```python
from build123d import *

# Parameters (mm, degrees)
CYLINDER039_R     = 68.3
CYLINDER039_DEPTH = 5
CYLINDER036_R     = 40
CYLINDER036_DEPTH = 27.4
CYLINDER035_R     = 45
CYLINDER035_DEPTH = 23.4
CYLINDER033_R     = 45
CYLINDER033_DEPTH = 25
CYLINDER032_R     = 48
CYLINDER032_DEPTH = 3.2
CYLINDER029_R     = 46.6
CYLINDER029_DEPTH = 6
CYLINDER038_R     = 46.6
CYLINDER038_DEPTH = 4
CYLINDER030_R     = 48
CYLINDER030_DEPTH = 4
CYLINDER037_R     = 48
CYLINDER037_DEPTH = 1.2
CYLINDER031_R     = 45
CYLINDER031_DEPTH = 25
CYLINDER034_R     = 51.3
CYLINDER034_DEPTH = 5
CHAMFER003_SIZE   = 1.2
CHAMFER002_SIZE   = 1.2


with BuildPart() as obj1:
    # Cylinder039 → Cylinder039 (new body)
    with BuildSketch(Plane.XY.offset(-23.2)):
        Circle(CYLINDER039_R)
    extrude(amount=CYLINDER039_DEPTH)


with BuildPart() as cone002:
    # Cone002 → Cone002 (revolve)
    with BuildSketch(Plane(origin=(0, 0, -15.2), x_dir=(-1, 0, 0), z_dir=(0, -1, 0))):
        Polygon((0, 0), (40, 0), (45, 5), (0, 5), align=None)
    revolve(axis=Axis((0, 0, -15.2), (0, 0, -1)))


with BuildPart() as fusion010:
    # Cylinder036 → Cylinder036 (new body)
    with BuildSketch(Plane.XY.offset(-17)):
        Circle(CYLINDER036_R)
    extrude(amount=CYLINDER036_DEPTH)

    # Fusion010: union Cone002
    add(cone002.part)


with BuildPart() as cut015:
    # Cylinder035 → Cylinder035 (new body)
    with BuildSketch(Plane.XY.offset(-20.2)):
        Circle(CYLINDER035_R)
    extrude(amount=CYLINDER035_DEPTH)

    # Cut015: cut Fusion010
    add(fusion010.part, mode=Mode.SUBTRACT)


with BuildPart() as cylinder033:
    # Cylinder033 → Cylinder033 (new body)
    with BuildSketch(Plane.XY.offset(-18)):
        Circle(CYLINDER033_R)
    extrude(amount=CYLINDER033_DEPTH)


with BuildPart() as cylinder032:
    # Cylinder032 → Cylinder032 (new body)
    with BuildSketch(Plane.XY):
        Circle(CYLINDER032_R)
    extrude(amount=CYLINDER032_DEPTH)


with BuildPart() as cylinder029:
    # Cylinder029 → Cylinder029 (new body)
    with BuildSketch(Plane.XY.offset(-14)):
        Circle(CYLINDER029_R)
    extrude(amount=CYLINDER029_DEPTH)


with BuildPart() as cylinder038:
    # Cylinder038 → Cylinder038 (new body)
    with BuildSketch(Plane.XY.offset(-4)):
        Circle(CYLINDER038_R)
    extrude(amount=CYLINDER038_DEPTH)


with BuildPart() as cylinder030:
    # Cylinder030 → Cylinder030 (new body)
    with BuildSketch(Plane.XY.offset(-8)):
        Circle(CYLINDER030_R)
    extrude(amount=CYLINDER030_DEPTH)


with BuildPart() as cut016:
    # Cylinder037 → Cylinder037 (new body)
    with BuildSketch(Plane.XY.offset(-15.2)):
        Circle(CYLINDER037_R)
    extrude(amount=CYLINDER037_DEPTH)

    # Fusion012: union Cylinder032, Cylinder029, Cylinder038, Cylinder030
    add(cylinder032.part)
    add(cylinder029.part)
    add(cylinder038.part)
    add(cylinder030.part)

    # Cut016: cut Cylinder033
    add(cylinder033.part, mode=Mode.SUBTRACT)


with BuildPart() as cylinder031:
    # Cylinder031 → Cylinder031 (new body)
    with BuildSketch(Plane.XY.offset(-23)):
        Circle(CYLINDER031_R)
    extrude(amount=CYLINDER031_DEPTH)


with BuildPart() as cut014:
    # Cylinder034 → Cylinder034 (new body)
    with BuildSketch(Plane.XY.offset(-20.2)):
        Circle(CYLINDER034_R)
    extrude(amount=CYLINDER034_DEPTH)

    # Cut017: cut Cylinder031
    add(cylinder031.part, mode=Mode.SUBTRACT)

    # Fusion009: union Cut016
    add(cut016.part)

    # Fusion011: union Cut015
    add(cut015.part)

    # Chamfer003
    chamfer003_edges = [cut014.edges().sort_by_distance(p)[0] for p in [
        (-46.6, 0, -14),
        (-46.6, 0, -4),
    ]]
    chamfer(chamfer003_edges, length=CHAMFER003_SIZE)

    # Chamfer002
    chamfer002_edges = [cut014.edges().sort_by_distance(p)[0] for p in [
        (-46.6, 0, -8),
        (-46.6, 0, 0),
    ]]
    chamfer(chamfer002_edges, length=CHAMFER002_SIZE)

    # Cut014: cut obj1
    add(obj1.part, mode=Mode.SUBTRACT)


solid = cut014.part
```
Here's how the part is built. I have some questions about the finished solid (model axes, mm). A direction names the side the tool comes from. Give positions to 0.01 mm unless a question says otherwise; leave off trailing zeros. Put each result on its own line as item: value. Start each with the question number.
(1) I need wall thicknesses on line 1 along Y through (x, z) = (0, -5); line 2 along Y through (x, z) = (34.5, -9.25). Which ranges of each line are inside material? Lowest first, please. Write a range as [from, to].
(2) Will these pins go through, and if not, where does the flat tip stop? pin 1 Ø10 at (x, z) = (-35, -2.5) entering from +Y; pin 2 Ø12 at (x, z) = (12.5, -14.5) entering from -Y; pin 3 Ø1.5 at (y, z) = (-40, -10.5) entering from -X.
(3) If we mould it in two halves opening along X, with no side actions, what happens to faces 4 (the flat face through (-18, 36, 3.2)), 5 (the cylindrical face through (-8.67, -39.05, -6.13)), 6 (the cylindrical face through (-47.954, 2.11, -6.028))? For each: +X half, -X half, draft (parallel to the pull), parting line (faces both ways), or undercut.
(4) For faces 1 (the flat face through (30, -38, -15.2)), 2 (the cylindrical face through (-6.678, 50.863, -16.721)), 3 (the cylindrical face through (-10.102, -45.492, -2.011)), which set-ups out of +Z, -Z, +X, -X, +Y, -Y let a thin tool reach every point of the face, with its end or its side?
Answer block:
1. line 1: [-48, -40], [40, 48]
1. line 2: [-31.33, -20.24], [20.24, 31.33]
2. pin 1: y = 37.28
2. pin 2: y = -50.88
2. pin 3: x = -25.12
3. face 4: draft
3. face 5: undercut
3. face 6: parting line
4. face 1: +Z
4. face 2: +Z, -Z
4. face 3: none
